Autodesk Inventor part; units mm, degrees
ref_plane "YZ Plane" through (0, 0, 0) normal (1, 0, 0) x (0, 1, 0)
ref_plane "XZ Plane" through (0, 0, 0) normal (0, 1, 0) x (-1, 0, 0)
ref_plane "XY Plane" through (0, 0, 0) normal (0, 0, 1) x (1, 0, 0)
sketch "Sketch1" plane through (0, 0, 0) normal (0, 1, 0) x (-1, 0, 0)
  line L0 (0, 0) -> (3.5814, 0)
  line L1 (3.5814, 0) -> (3.5814, -9.017)
  line L2 (3.5814, -9.017) -> (0, -9.017)
  line L3 (0, -9.017) -> (0, 0)
  dimension "d0" = 3.5814
  dimension "d1" = 9.017
extrude "Extrusion1" add sketch "Sketch1" along normal blind 6.35
sketch "Sketch2" plane through (0, 6.35, 0) normal (0, 1, 0) x (1, 0, 0)
  line L0 (-2.6162, 2.5908) -> (-1.1684, 2.5908)
  line L1 (-1.1684, 2.5908) -> (-1.1684, 4.0386)
  line L2 (-1.1684, 4.0386) -> (-2.6162, 4.0386)
  line L3 (-2.6162, 4.0386) -> (-2.6162, 2.5908)
  line L4 (-3.5814, 0) -> (0, 0)
  line L5 (0, 0) -> (0, 9.017)
  dimension "d4" = 1.4478
  dimension "d5" = 1.4478
  dimension "d6" = 2.5908
  dimension "d7" = 1.1684
extrude "Extrusion2" add sketch "Sketch2" along normal blind 2.159
properties part number "switch"
Model file for the job. Use its own axes, mm. A direction names the side the tool comes from. Round coordinates to 2 decimals unless told otherwise and drop trailing zeros. Order: outer loops, then holes, each group sorted by start corner. A loop starts at its lowest first (then second) coordinate and runs counter-clockwise, first axis right, second up. Notation, with made-up numbers: M 87.25,30.25 L 114.25,30.25 A24 ccw 114.25,45.25 Z; hole C 6.25,76.5 d10. An arc over 180 degrees is marked long. Write each question's results on one line, items separated by ' | '. Start each with the question number.
(1) Saw through at A-A, the plane z = -3. Give the cut face in (x, y), then the cut area to 3 significant figures.
(2) Drop flat-ended pins along their axis: pin 1 (1.2 mm diameter, centred on y = 8, z = -3.5, fed in from -X); pin 2 (2 mm diameter, centred on x = -1.5, y = 7, fed in from -Z); pin 3 (1.8 mm diameter, centred on x = -1.5, z = -5, fed in from +Y). Give the stop position or say it passes through.
(3) Which spindle directions (+Z, -Z, +X, -X, +Y, -Y) get a long thin tool onto all of the face, cutting with end or side? Do faces 1 (the face through (-2, 7, -2.591)), 2 (the face through (-2, 7, -4.039)), 3 (the face through (-2.616, 7, -3)), 4 (the face through (-1.168, 7, -3)). Say none if no direction does.
(4) Probe probe 1 along Y at (x, z) = (-3.3, -2); probe 2 along Z at (x, y) = (-1.75, 6.5). List the from-to ranges inside material, lowest first. Write a range as from..to.
(5) Saw through at B-B, the plane x = -1.5. Give the cut face in (y, z), then the cut area to 3 significant figures.
(6) Saw through at D-D, the plane z = -7. Give the cut face in (x, y), then the cut area to 3 significant figures.
(7) Saw through at C-C, the plane x = -3.3. Give the cut face in (y, z).
Established:
1) outline: M -3.58,0 L 0,0 L 0,6.35 L -1.17,6.35 L -1.17,8.51 L -2.62,8.51 L -2.62,6.35 L -3.58,6.35 Z | area: 25.9 mm^2
2) pin 1: stops at x = -2.62 | pin 2: stops at z = -9.02 | pin 3: stops at y = 6.35
3) face 1: +Z, +X, -X, +Y | face 2: -Z, +X, -X, +Y | face 3: +Z, -Z, -X, +Y | face 4: +Z, -Z, +X, +Y
4) probe 1: y = 0..6.35 | probe 2: z = -4.04..-2.59
5) outline: M 0,-9.02 L 6.35,-9.02 L 6.35,-4.04 L 8.51,-4.04 L 8.51,-2.59 L 6.35,-2.59 L 6.35,0 L 0,0 Z | area: 60.4 mm^2
6) outline: M -3.58,0 L 0,0 L 0,6.35 L -3.58,6.35 Z | area: 22.7 mm^2
7) outline: M 0,-9.02 L 6.35,-9.02 L 6.35,0 L 0,0 Z
